The listing builds one solid part. Answer for the finished solid, in the listing's coordinates (mm). A direction names the side the tool comes from. Coordinates: 2 decimals unless noted, no trailing zeros. Write each loop counter-clockwise with the first axis right and the second up, starting at its lowest first coordinate (ties: lowest second). Pieces come first, ordered by that corner, then holes.
(1) Which of the six approach directions +Z, -Z, +X, -X, +Y, -Y give full straight-line access (tool end or side, diameter ignored) to faces 5 (the flat face through (0, 166, 22.5)), 6 (the flat face through (0, 158, 17.5)), 7 (the flat face through (-22.5, 186, 0)), 8 (the flat face through (0, 214.039, 20)), 9 (the flat face through (22.5, 186, 0))?
(2) Straight lines are drawn through the part: line 1 (Z direction, x = 25, y = 97.45); line 2 (X direction, y = 244, z = 21.5). For each, find the intervals that lie inside material, in ascending order.
(3) The part is cut by section A-A on x = 2. Determine the outline of the cut face in (y, z), plus the area to 3 significant figures.
(4) The part is cut by section C-C on z = -14. Determine the outline of the cut face in (x, y), plus the area to 3 significant figures.
(5) The part is cut by section D-D on y = 227. Determine the outline of the cut face in (x, z), plus the area to 3 significant figures.
(6) Given P1, Ø10.5, axis at x = -2.5, y = 161.5, coming from the +Z side; P2, Ø5, axis at x = 1, z = 3, coming from the +Y side; P3, Ø1, axis at y = 164.5, z = -3, coming from the -X side; P4, Ø2.5, axis at x = 25, z = 25, coming from the -Y side, each flat-ended and moving along its own axis, determine where each tip first touches the part or whether it passes through.
(7) For a pull along Y with two mould halves and no side action, classify faces 1 (the flat face through (0, 272, -17.5)), 2 (the flat face through (20, 273.612, 0)), 3 (the flat face through (0, 270.587, -20)), 4 (the flat face through (0, 249.413, -20)) as +Y half, -Y half, draft (parallel to the pull), parting line (faces both ways), or undercut.
(8) The part is cut by section B-B on y = 107. Determine the outline of the cut face in (x, z).
from build123d import *

# Parameters (mm, degrees)
CROQUIS1_W                 = 45
CROQUIS1_H                 = 45
SALIENTE_EXTRUIR1_DEPTH    = 300
CROQUIS4_W                 = 18
CROQUIS4_H                 = 34
CORTAR_EXTRUIR2_DEPTH      = 46
CROQUIS8_W                 = 35
CROQUIS8_H                 = 35
CORTAR_EXTRUIR3_DEPTH      = 301
CROQUIS9_W                 = 35
CROQUIS9_H                 = 21.174410022
CORTAR_EXTRUIR4_DEPTH      = 10
CROQUIS10_R                = 1
CORTAR_EXTRUIR5_DEPTH      = 10
CROQUIS17_W                = 35
CROQUIS17_H                = 54.573397986
CORTAR_EXTRUIR9_DEPTH      = 10
CROQUIS11_W                = 45
CROQUIS11_H                = 26.387879272
CORTAR_EXTRUIR6_DEPTH      = 46
CROQUIS13_W                = 45
CROQUIS13_H                = 100
CORTAR_EXTRUIR7_DEPTH      = 23.5
CORTAR_EXTRUIR7_DEPTH_BACK = 23.5
CROQUIS14_W                = 55
CROQUIS14_H                = 55
SALIENTE_EXTRUIR2_DEPTH    = 5
CROQUIS16_R                = 1
CORTAR_EXTRUIR8_DEPTH      = 1
CORTAR_EXTRUIR8_DEPTH_BACK = 179.612120728


with BuildPart() as part:
    # Croquis1 → Saliente-Extruir1 (new body)
    with BuildSketch(Plane(origin=(0, 0, 0), x_dir=(1, 0, 0), z_dir=(0, 1, 0))):
        Rectangle(CROQUIS1_W, CROQUIS1_H)
    extrude(amount=SALIENTE_EXTRUIR1_DEPTH)

    # Croquis4 → Cortar-Extruir2 (cut, through all)
    with BuildSketch(Plane.ZY.offset(22.5)):
        with Locations((13.5, 17)):
            Rectangle(CROQUIS4_W, CROQUIS4_H)
    extrude(amount=-CORTAR_EXTRUIR2_DEPTH, mode=Mode.SUBTRACT)

    # Croquis8 → Cortar-Extruir3 (cut, through all)
    with BuildSketch(Plane(origin=(0, 300, 0), x_dir=(1, 0, 0), z_dir=(0, 1, 0))):
        Rectangle(CROQUIS8_W, CROQUIS8_H)
    extrude(amount=-CORTAR_EXTRUIR3_DEPTH, mode=Mode.SUBTRACT)

    # Croquis9 → Cortar-Extruir4 (cut)
    with BuildSketch(Plane(origin=(0, 0, -22.5), x_dir=(-1, 0, 0), z_dir=(0, 0, -1))):
        with Locations((0, 260)):
            Rectangle(CROQUIS9_W, CROQUIS9_H)
    extrude(amount=-CORTAR_EXTRUIR4_DEPTH, mode=Mode.SUBTRACT)

    # Croquis10 → Cortar-Extruir5 (cut)
    with BuildSketch(Plane.XY.offset(22.5)):
        with Locations((0, 260)):
            Circle(CROQUIS10_R)
    extrude(amount=-CORTAR_EXTRUIR5_DEPTH, mode=Mode.SUBTRACT)

    # Croquis17 → Cortar-Extruir9 (cut)
    with BuildSketch(Plane.XY.offset(22.5)):
        with Locations((0, 241.325421735)):
            Rectangle(CROQUIS17_W, CROQUIS17_H)
    extrude(amount=-CORTAR_EXTRUIR9_DEPTH, mode=Mode.SUBTRACT)

    # Croquis11 → Cortar-Extruir6 (cut, through all)
    with BuildSketch(Plane.XY.offset(22.5)):
        with Locations((0, 286.806060364)):
            Rectangle(CROQUIS11_W, CROQUIS11_H)
    extrude(amount=-CORTAR_EXTRUIR6_DEPTH, mode=Mode.SUBTRACT)

    # Croquis13 → Cortar-Extruir7 (cut, two sides)
    with BuildSketch(Plane(origin=(0, 0, 0), x_dir=(0, 0, -1), z_dir=(1, 0, 0))) as cortar_extruir7_sk:
        with Locations((0, 50)):
            Rectangle(CROQUIS13_W, CROQUIS13_H)
    extrude(amount=CORTAR_EXTRUIR7_DEPTH, mode=Mode.SUBTRACT)
    extrude(cortar_extruir7_sk.sketch, amount=-CORTAR_EXTRUIR7_DEPTH_BACK, mode=Mode.SUBTRACT)

    # Croquis14 → Saliente-Extruir2 (add)
    with BuildSketch(Plane.XZ.offset(-100)):
        Rectangle(CROQUIS14_W, CROQUIS14_H)
    extrude(amount=SALIENTE_EXTRUIR2_DEPTH)

    # Croquis16 → Cortar-Extruir8 (cut, two sides)
    with BuildSketch(Plane.XZ.offset(-95)) as cortar_extruir8_sk:
        with Locations((25, 25)):
            Circle(CROQUIS16_R)
        with Locations((-25, 25)):
            Circle(CROQUIS16_R)
        with Locations((-25, -25)):
            Circle(CROQUIS16_R)
        with Locations((25, -25)):
            Circle(CROQUIS16_R)
    extrude(amount=CORTAR_EXTRUIR8_DEPTH, mode=Mode.SUBTRACT)
    extrude(cortar_extruir8_sk.sketch, amount=-CORTAR_EXTRUIR8_DEPTH_BACK, mode=Mode.SUBTRACT)


solid = part.part
Model answer:
1. face 5: +Z, +X, -X, +Y
1. face 6: +Y
1. face 7: +Z, -Z, -X, +Y
1. face 8: +Z
1. face 9: +Z, -Z, +X, +Y
2. line 1: z = -27.5 to -26, -24 to 24, 26 to 27.5
2. line 2: x = -22.5 to -17.5, 17.5 to 22.5
3. outline: (95, -27.5) - (100, -27.5) - (100, -22.5) - (249.41, -22.5) - (249.41, -17.5) - (100, -17.5) - (100, 17.5) - (214.04, 17.5) - (214.04, 22.5) - (100, 22.5) - (100, 27.5) - (95, 27.5) - close; (268.61, 17.5) - (273.61, 17.5) - (273.61, 22.5) - (268.61, 22.5) - close; (270.59, -22.5) - (273.61, -22.5) - (273.61, -17.5) - (270.59, -17.5) - close
3. area: 1,630 mm2
4. outline: (-27.5, 95) - (27.5, 95) - (27.5, 100) - (22.5, 100) - (22.5, 273.61) - (17.5, 273.61) - (17.5, 100) - (-17.5, 100) - (-17.5, 273.61) - (-22.5, 273.61) - (-22.5, 100) - (-27.5, 100) - close
4. area: 2,010 mm2
5. outline: (-22.5, -22.5) - (22.5, -22.5) - (22.5, 22.5) - (17.5, 22.5) - (17.5, -17.5) - (-17.5, -17.5) - (-17.5, 22.5) - (-22.5, 22.5) - close
5. area: 625 mm2
6. P1: stops at z = 22.5
6. P2: stops at y = 100
6. P3: stops at x = -22.5
6. P4: stops at y = 95
7. face 1: draft
7. face 2: +Y half
7. face 3: undercut
7. face 4: undercut
8. outline: (-22.5, -22.5) - (22.5, -22.5) - (22.5, 22.5) - (-22.5, 22.5) - close; hole (-17.5, -17.5) - (17.5, -17.5) - (17.5, 17.5) - (-17.5, 17.5) - close
